Check sheet for the modelled part. Datum: model origin and axes. Units: mm. Round coordinates to 2 decimals unless told otherwise and drop trailing zeros. Write each loop counter-clockwise with the first axis right and the second up, starting at its lowest first coordinate (ties: lowest second). Pieces come first, ordered by that corner, then holes. Notation, with made-up numbers: M 47.25,63 L 99.25,63 A4 ccw 99.25,68 Z; hole C 87,-7 d3. An arc over 180 degrees is marked long. One line per item, written item: value.
from build123d import *

# Parameters (mm, degrees)
SKETCH1_R           = 2
BOSS_EXTRUDE1_DEPTH = 10
SKETCH2_R           = 9.5
CUT_EXTRUDE1_DEPTH  = 6
SKETCH3_R           = 5
CUT_EXTRUDE2_DEPTH  = 11
CUT_EXTRUDE3_DEPTH  = 11


with BuildPart() as part:
    # Sketch1 → Boss-Extrude1 (new body)
    with BuildSketch(Plane(origin=(0, 0, 0), x_dir=(1, 0, 0), z_dir=(0, 1, 0))):
        with BuildLine():
            Line((0, 11.5), (250, 11.5))
            ThreePointArc((250, 11.5), (261.5, 0), (250, -11.5))
            Line((250, -11.5), (0, -11.5))
            ThreePointArc((0, -11.5), (-11.5, 0), (0, 11.5))
        make_face()
        Circle(SKETCH1_R, mode=Mode.SUBTRACT)
    extrude(amount=BOSS_EXTRUDE1_DEPTH)

    # Sketch2 → Cut-Extrude1 (cut)
    with BuildSketch(Plane(origin=(0, 10, 0), x_dir=(1, 0, 0), z_dir=(0, 1, 0))):
        with Locations((250, 0)):
            Circle(SKETCH2_R)
    extrude(amount=-CUT_EXTRUDE1_DEPTH, mode=Mode.SUBTRACT)

    # Sketch3 → Cut-Extrude2 (cut, through all)
    with BuildSketch(Plane(origin=(0, 0, 0), x_dir=(-1, 0, 0), z_dir=(0, -1, 0))):
        with Locations((-250, 0)):
            Circle(SKETCH3_R)
    extrude(amount=-CUT_EXTRUDE2_DEPTH, mode=Mode.SUBTRACT)

    # Sketch4 → Cut-Extrude3 (cut, through all)
    with BuildSketch(Plane(origin=(0, 10, 0), x_dir=(1, 0, 0), z_dir=(0, 1, 0))):
        with BuildLine():
            Line((18, 6.5), (116, 6.5))
            ThreePointArc((116, 6.5), (122.5, 0), (116, -6.5))
            Line((116, -6.5), (18, -6.5))
            ThreePointArc((18, -6.5), (11.5, 0), (18, 6.5))
        make_face()
        with BuildLine():
            Line((134, 6.5), (232, 6.5))
            ThreePointArc((232, 6.5), (238.5, 0), (232, -6.5))
            Line((232, -6.5), (134, -6.5))
            ThreePointArc((134, -6.5), (127.5, 0), (134, 6.5))
        make_face()
    extrude(amount=-CUT_EXTRUDE3_DEPTH, mode=Mode.SUBTRACT)


solid = part.part
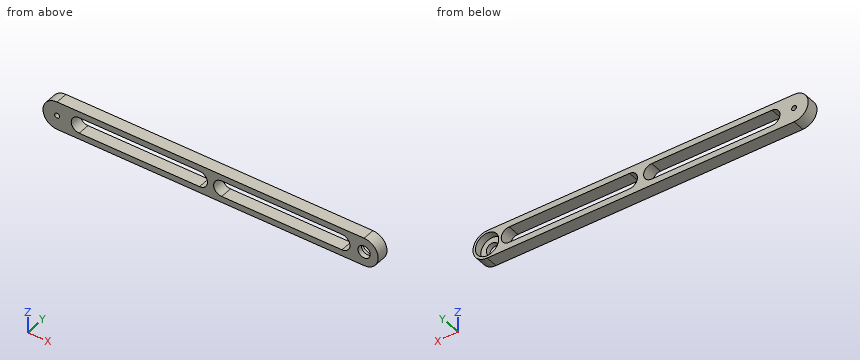
Q1. Sectioned sample at B-B on x = 144. Enter the section's corners in (y, z).
Completed:
outline: M 0,-11.5 L 10,-11.5 L 10,-6.5 L 0,-6.5 Z; M 0,6.5 L 10,6.5 L 10,11.5 L 0,11.5 Z
Q2. Depth check by flat-ended pin: P1, Ø1.5, axis at y = 3.5, z = 6, coming from the -X side; P2, Ø11.5, axis at x = 250, z = 0, coming from the -Y side; P3, Ø1, axis at y = 1, z = 3, coming from the -X side (3 decimals); P4, Ø6, axis at y = 5, z = 6.5, coming from the +X side. Enter the tip coordinate at first touch or a pass-through.
Completed:
P1: x = -10.23
P2: y = 0
P3: x = -11.225
P4: x = 260.95
Q3. Sectioned sample at A-A on y = 6. Enter the section's corners in (x, z).
Completed:
outline: M 0,-11.5 L 250,-11.5 A11.5 ccw 250,11.5 L 0,11.5 A11.5 ccw Z; hole C 0,0 d4; hole M 18,-6.5 L 116,-6.5 A6.5 ccw 116,6.5 L 18,6.5 A6.5 ccw Z; hole M 134,-6.5 L 232,-6.5 A6.5 ccw 232,6.5 L 134,6.5 A6.5 ccw Z; hole C 250,0 d19
Q4. Scan lines: line 1 (X direction, y = 3, z = 0); line 2 (X direction, y = 8.4, z = 0); line 3 (Z direction, x = 250, y = 5.4). Record each from-to range of solid material in increasing order. Write a range as [from, to].
Completed:
line 1: [-11.5, -2], [2, 11.5], [122.5, 127.5], [238.5, 245], [255, 261.5]
line 2: [-11.5, -2], [2, 11.5], [122.5, 127.5], [238.5, 240.5], [259.5, 261.5]
line 3: [-11.5, -9.5], [9.5, 11.5]
